The listing builds one solid part. Answer for the finished solid, in the listing's coordinates (mm). A direction names the side the tool comes from. Coordinates: 2 decimals unless noted, no trailing zeros. Write each loop counter-clockwise with the first axis right and the second up, starting at its lowest first coordinate (ties: lowest second). Pieces come first, ordered by that corner, then holes. Notation, with made-up numbers: M -20.75,65 L 22.25,65 A14 ccw 22.25,75 Z; hole C -31.5,19.5 d2. An arc over 180 degrees is marked long. Answer as CSV lines item,"result".
```python
from build123d import *

# Parameters (mm, degrees)
SZKIC1_R                               = 21
DODANIE_WYCI_GNI_CIE1_DEPTH            = 10
SZKIC2_R                               = 12.5
DODANIE_WYCI_GNI_CIE2_DEPTH            = 15
OTWORY_USTALAJ_CE_5_0MM1_D             = 5
SZYK_KO_OWY1_COUNT                     = 6
WYTNIJ_WYCI_GNI_CIE1_REACH             = 40.82
SZKIC8_R                               = 5
WYTNIJ_WYCI_GNI_CIE1_DIRECTION_2_DEPTH = 39.820097888


with BuildPart() as part:
    # Szkic1 → Dodanie-wyciągnięcie1 (new body)
    with BuildSketch(Plane.XY):
        Circle(SZKIC1_R)
    extrude(amount=DODANIE_WYCI_GNI_CIE1_DEPTH)

    # Szkic2 → Dodanie-wyciągnięcie2 (add)
    with BuildSketch(Plane.XY.offset(10)):
        Circle(SZKIC2_R)
    extrude(amount=DODANIE_WYCI_GNI_CIE2_DEPTH)

    # Otwory ustalające Ø5.0mm1 (through all)
    with Locations(Plane.XY.offset(10)):
        with Locations((0, 17)):
            otwory_ustalaj_ce_5_0mm1 = Hole(OTWORY_USTALAJ_CE_5_0MM1_D / 2)

    # Szyk kołowy1: Otwory ustalające Ø5.0mm1 ×6 about axis
    szyk_ko_owy1_axis = Axis((0, 0, 0), (0, 0, 1))
    for i in range(1, SZYK_KO_OWY1_COUNT):
        add(otwory_ustalaj_ce_5_0mm1.rotate(szyk_ko_owy1_axis, i * 360 / SZYK_KO_OWY1_COUNT), mode=Mode.SUBTRACT)

    # Szkic8 → Wytnij-wyciągnięcie1 (cut, up to next)
    with BuildSketch(Plane.XY.offset(25), mode=Mode.PRIVATE) as wytnij_wyci_gni_cie1_sk1:
        with Locations(Location((0, 0, 0), (0, 0, 180))):
            Circle(SZKIC8_R)
    wytnij_wyci_gni_cie1_tool1 = extrude(wytnij_wyci_gni_cie1_sk1.sketch, amount=-WYTNIJ_WYCI_GNI_CIE1_REACH, mode=Mode.PRIVATE) & part.part
    add(wytnij_wyci_gni_cie1_tool1.solids().sort_by_distance((0, 0, 25))[0], mode=Mode.SUBTRACT)

    # Szkic8 → Wytnij-wyciągnięcie1 direction 2 (cut)
    with BuildSketch(Plane.XY.offset(25)):
        with Locations(Location((0, 0, 0), (0, 0, 180))):
            Circle(SZKIC8_R)
    extrude(amount=WYTNIJ_WYCI_GNI_CIE1_DIRECTION_2_DEPTH, mode=Mode.SUBTRACT)


solid = part.part
```
Q1. Flat-ended cylindrical pins translate along their axes: pin 1 Ø1.5 at (x, z) = (-7, 3) entering from -Y; pin 2 Ø3 at (x, y) = (-14.72, -8.5) entering from +Z; pin 3 Ø5 at (x, z) = (8, 3) entering from -Y; pin 4 Ø3 at (x, z) = (11, 18.5) entering from +Y. Find the tip coordinate at first contact, or state that the pin passes through.
Output:
pin 1,"y = -20.05"
pin 2,"through"
pin 3,"y = -20.27"
pin 4,"y = 8.12"
Q2. Straight lines are drawn through the part: line 1 (Y direction, x = 0, z = 6.25); line 2 (Z direction, x = -15.5, y = 11); line 3 (X direction, y = 16.5, z = 1). For each, find the intervals that lie inside material, in ascending order.
Output:
line 1,"-21 to -19.5, -14.5 to -5, 5 to 14.5, 19.5 to 21"
line 2,"0 to 10"
line 3,"-12.99 to -2.45, 2.45 to 12.99"
Q3. Find section B-B (y = 0). Give the vertices of the cut face in (x, z), and give its area (3 significant figures).
Output:
outline,"M -21,0 L -5,0 L -5,25 L -12.5,25 L -12.5,10 L -21,10 Z; M 5,0 L 21,0 L 21,10 L 12.5,10 L 12.5,25 L 5,25 Z"
area,"545 mm2"
Q4. For faces 5 (the cylindrical face through (14.18, 10.94, 4.93)), 6 (the flat face through (9, -9, 10)), determine the directions among +Z, -Z, +X, -X, +Y, -Y from which every point of the face is accessible in a straight line to the end or side of a thin tool.
Output:
face 5,"+Z, -Z"
face 6,"+Z"
Q5. The mould has two halves that part along X. Classify faces 1 (the cylindrical face through (1.34, -19.11, 4.93)), 2 (the cylindrical face through (11.923, 3.755, 17.395)), 3 (the flat face through (-0.2, -5.4, 25)), 4 (the cylindrical face through (5, 0, 13)): pulls with the +X half, pulls with the -X half, needs draft (parallel to the pull), parting line crosses it, or undercut.
Output:
face 1,"undercut"
face 2,"parting line crosses it"
face 3,"needs draft"
face 4,"undercut"
Q6. Find section D-D (y = -8.5). Give the vertices of the cut face in (x, z), and give its area (3 significant figures).
Output:
outline,"M -19.2,0 L -17.22,0 L -17.22,10 L -19.2,10 Z; M -12.22,0 L 12.22,0 L 12.22,10 L 9.17,10 L 9.17,25 L -9.17,25 L -9.17,10 L -12.22,10 Z; M 17.22,0 L 19.2,0 L 19.2,10 L 17.22,10 Z"
area,"559 mm2"
Q7. Find section C-C (x = 0). Give the vertices of the cut face in (y, z).
Output:
outline,"M -21,0 L -19.5,0 L -19.5,10 L -21,10 Z; M -14.5,0 L -5,0 L -5,25 L -12.5,25 L -12.5,10 L -14.5,10 Z; M 5,0 L 14.5,0 L 14.5,10 L 12.5,10 L 12.5,25 L 5,25 Z; M 19.5,0 L 21,0 L 21,10 L 19.5,10 Z"
Q8. Find section A-A (x = 16.5). Give the vertices of the cut face in (y, z).
Output:
outline,"M -12.99,0 L -10.26,0 L -10.26,10 L -12.99,10 Z; M -6.74,0 L 6.74,0 L 6.74,10 L -6.74,10 Z; M 10.26,0 L 12.99,0 L 12.99,10 L 10.26,10 Z"
